from build123d import *

# Parameters (mm, degrees)
SKETCH_1_R          = 1.35
EXTRUDE_1_DEPTH     = 40
EXTRUDE_2_DEPTH     = 10
SKETCH_3_W          = 36
SKETCH_3_H          = 37.441664415
SKETCH_3_R          = 11
EXTRUDE_3_DEPTH     = 5
SKETCH_7_W          = 36
SKETCH_7_H          = 37.441664415
CUT_EXTRUDE_4_DEPTH = 5
CUT_EXTRUDE_START   = -12
SKETCH_8_R          = 1.35
CUT_EXTRUDE_5_DEPTH = 12
SKETCH_10_R         = 1.34
SKETCH_10_R_2       = 1.35
CUT_EXTRUDE_6_DEPTH = 52


with BuildPart() as part:
    # 草图1 → 凸台-拉伸1 (new body)
    with BuildSketch(Plane.XY):
        with BuildLine():
            Line((-10, -4), (10, -4))
            ThreePointArc((10, -4), (13.795550466, -1.262456597), (12.395858862, 3.203101671))
            Line((12.395858862, 3.203101671), (6.347732719, 7.726984491))
            Line((6.347732719, 7.726984491), (0, 7.726984491))
            Line((0, 7.726984491), (-6.347732719, 7.726984491))
            Line((-6.347732719, 7.726984491), (-12.395858862, 3.203101671))
            ThreePointArc((-12.395858862, 3.203101671), (-13.795550466, -1.262456597), (-10, -4))
        make_face()
        with Locations((10, 0)):
            Circle(SKETCH_1_R, mode=Mode.SUBTRACT)
        with Locations((-10, 0)):
            Circle(SKETCH_1_R, mode=Mode.SUBTRACT)
    extrude(amount=EXTRUDE_1_DEPTH)

    # 草图2 → 凸台-拉伸2 (add)
    with BuildSketch(Plane.XZ.offset(4)):
        Polygon((-10, 37.441664415), (-18, 37.441664415), (-18, 0), (0, 0), (10, 0), (18, 0), (18, 37.441664415), align=None)
    extrude(amount=-EXTRUDE_2_DEPTH)

    # 草图3 → 凸台-拉伸3 (add)
    with BuildSketch(Plane.XZ.offset(4)):
        with Locations((0, 18.720832208)):
            Rectangle(SKETCH_3_W, SKETCH_3_H)
        with Locations(Location((0, 16, 0), (0, 0, 270))):
            Circle(SKETCH_3_R, mode=Mode.SUBTRACT)
    extrude(amount=EXTRUDE_3_DEPTH)

    # 草图7 → 切除-拉伸4 (cut)
    with BuildSketch(Plane.XZ.offset(9)):
        with Locations((0, 18.720832208)):
            Rectangle(SKETCH_7_W, SKETCH_7_H)
    extrude(amount=-CUT_EXTRUDE_4_DEPTH, mode=Mode.SUBTRACT)

    # 草图8 → 切除-拉伸5 (cut)
    with BuildSketch(Plane.XY.offset(37.441664415).offset(CUT_EXTRUDE_START)):
        with Locations((10, 0)):
            Circle(SKETCH_8_R)
        with Locations((-10, 0)):
            Circle(SKETCH_8_R)
    extrude(amount=CUT_EXTRUDE_5_DEPTH, mode=Mode.SUBTRACT)

    # 草图10 → 切除-拉伸6 (cut)
    with BuildSketch(Plane(origin=(0, 0, 0), x_dir=(-1, 0, 0), z_dir=(0, 0, -1))):
        with Locations((10, 0)):
            Circle(SKETCH_10_R)
        with Locations((-10, 0)):
            Circle(SKETCH_10_R_2)
    extrude(amount=-CUT_EXTRUDE_6_DEPTH, mode=Mode.SUBTRACT)


solid = part.part
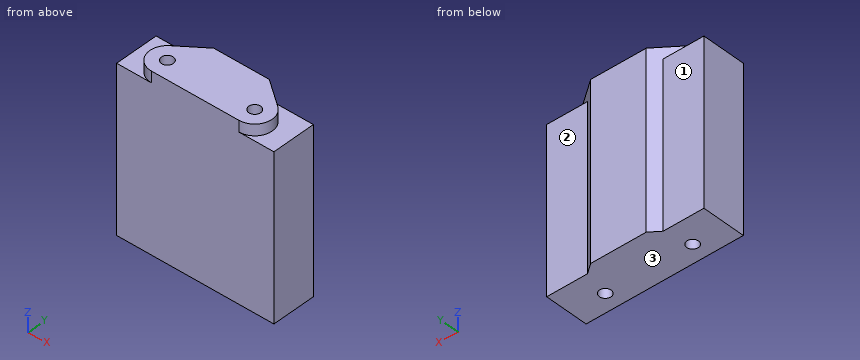
Work out the finished part from the listing and answer in its coordinate system (mm). Face numbers are marked on the shaded views. A direction names the side the tool comes from. Give positions to 0.01 mm unless a question says otherwise; leave off trailing zeros. Order: outer loops, then holes, each group sorted by start corner. A loop starts at its lowest first (then second) coordinate and runs counter-clockwise, first axis right, second up. Notation, with made-up numbers: (41.5, 26) -> (96.5, 26) arc R33 cw to (96.5, 55) -> close; hole circle Ø8 at (49.5, 38). An arc over 180 degrees is marked (long way). One line per item, written item: value.
Item 1: Find section A-A, the plane y = 0. State how many separate pieces and enclosed holes the cut face has, plus the area to 3 significant figures.
Answer sheet:
separate pieces: 3
enclosed holes: 0
area: 1,200 mm²
Item 2: Straight lines are drawn through the part: probe 1 along Y at (x, z) = (-10, 33.5); probe 2 along X at (y, z) = (-1, 29.5); probe 3 along X at (y, z) = (0.75, 21.5). For each, find the intervals that lie inside material, in ascending order.
Answer sheet:
probe 1: -4 to -1.35, 1.35 to 6
probe 2: -18 to -10.91, -9.09 to 9.09, 10.91 to 18
probe 3: -18 to -11.11, -8.89 to 8.88, 11.12 to 18
Item 3: Find section D-D, the plane x = -8. Give the vertices of the cut face in (y, z), plus the area to 3 significant figures.
Answer sheet:
outline: (-4, 0) -> (6.49, 0) -> (6.49, 40) -> (-4, 40) -> close
area: 420 mm²
Item 4: Find section C-C, the plane z = 29.5. Give the vertices of the cut face in (x, y), plus the area to 3 significant figures.
Answer sheet:
outline: (-18, -4) -> (18, -4) -> (18, 6) -> (8.66, 6) -> (6.35, 7.73) -> (-6.35, 7.73) -> (-8.66, 6) -> (-18, 6) -> close; hole circle Ø2.7 at (-10, 0); hole circle Ø2.7 at (10, 0)
area: 374 mm²
Item 5: Flat-ended cylindrical pins translate along their axes: P1, Ø7.5, axis at x = 12, z = 11, coming from the +Y side; P2, Ø2.5, axis at x = 10, y = 0, coming from the +Z side; P3, Ø10.5, axis at x = -14, z = 24.5, coming from the +Y side. Find the tip coordinate at first contact, or state that the pin passes through.
Answer sheet:
P1: y = 6.3
P2: through
P3: y = 6
Item 6: Find section B-B, the plane z = 20. Give the vertices of the cut face in (x, y).
Answer sheet:
outline: (-18, -4) -> (18, -4) -> (18, 6) -> (8.66, 6) -> (6.35, 7.73) -> (-6.35, 7.73) -> (-8.66, 6) -> (-18, 6) -> close; hole circle Ø2.68 at (-10, 0); hole circle Ø2.7 at (10, 0)
Item 7: A tool of negligible diameter and unlimited length cuts with its end or side. For the marked faces 1, 2 and 3, from which of +Z, -Z, +X, -X, +Y, -Y can it reach the whole face along a straight path? Write none if from no direction.
Answer sheet:
face 1: +Z, -Z, -X, +Y
face 2: +Z, -Z, +X, +Y
face 3: -Z, +X, -X, +Y, -Y
